Model file for the job. Use its own axes, mm. A direction names the side the tool comes from. Round coordinates to 2 decimals unless told otherwise and drop trailing zeros. Order: outer loops, then holes, each group sorted by start corner. A loop starts at its lowest first (then second) coordinate and runs counter-clockwise, first axis right, second up. Notation, with made-up numbers: (51, 50) - (94, 50) arc R37 ccw to (94, 86) - close; hole circle Ø4 at (44.5, 60). An arc over 180 degrees is marked (long way). Put each result on its own line as item: value. Start each with the question number.
Item 1: Probe probe 1 along Z at (x, y) = (0, 7); probe 2 along Z at (x, y) = (-22.5, 4.5); probe 3 along X at (y, z) = (3, 5). List the from-to ranges inside material, lowest first.
Item 2: Pin check, flat tips, straight feed: pin 1 Ø3 at (y, z) = (4, 2) entering from +X; pin 2 Ø3.5 at (x, y) = (-21, 6) entering from +Z; pin 3 Ø2 at (x, y) = (8.5, 4) entering from -Z. Stop position of each tip, or through.
Item 3: Saw through at A-A on z = 0. List the corners of the cut face in (x, y).
Item 4: Saw through at B-B on y = 3.5. List the corners of the cut face in (x, z).
Item 5: Mould opens along X. For faces 1 (the face through (9.83, 4.93, -37.74)), 2 (the face through (-29, 4, 0)), 3 (the face through (-14, 0, -27)), 4 (the face through (-23.54, 4.44, 16.94)) say: pulls with the +X half, pulls with the -X half, needs draft (parallel to the pull), parting line crosses it, or undercut.
Item 6: Which spindle directions (+Z, -Z, +X, -X, +Y, -Y) get a long thin tool onto all of the face, cutting with end or side? Do faces 5 (the face through (23.54, 4.44, -16.94)), 6 (the face through (9.56, 10.48, -28.94)). Say none if no direction does.
```python
from build123d import *

# Parameters (mm, degrees)
SKETCH1_R           = 39
BOSS_EXTRUDE1_DEPTH = 12
FILLET1_R           = 2
CHAMFER1_SIZE       = 3
SKETCH2_W           = 43
SKETCH2_H           = 43
CUT_EXTRUDE2_DEPTH  = 57.444663167


with BuildPart() as part:
    # Sketch1 → Boss-Extrude1 (new body)
    with BuildSketch(Plane(origin=(0, 0, 0), x_dir=(1, 0, 0), z_dir=(0, 1, 0))):
        with Locations(Location((0, 0, 0), (0, 0, 270))):
            Circle(SKETCH1_R)
        Polygon((17.922985674, 24.668873442), (0, 30.492404503), (-17.922985674, 24.668873442), (-29, 9.422671191), (-29, -9.422671191), (-17.922985674, -24.668873442), (0, -30.492404503), (17.922985674, -24.668873442), (29, -9.422671191), (29, 9.422671191), align=None, mode=Mode.SUBTRACT)
    extrude(amount=BOSS_EXTRUDE1_DEPTH)

    # Fillet1
    fillet1_edges = [part.edges().sort_by_distance(p)[0] for p in [
        (0, 12, -39),
    ]]
    fillet(fillet1_edges, radius=FILLET1_R)

    # Chamfer1
    chamfer1_edges = [part.edges().sort_by_distance(p)[0] for p in [
        (23.461492837, 12, -17.045772316),
        (8.961492837, 12, -27.580638973),
        (-8.961492837, 12, -27.580638973),
        (-23.461492837, 12, -17.045772316),
        (-29, 12, 0),
        (-23.461492837, 12, 17.045772316),
        (-8.961492837, 12, 27.580638973),
        (8.961492837, 12, 27.580638973),
        (23.461492837, 12, 17.045772316),
        (29, 12, 0),
    ]]
    chamfer(chamfer1_edges, length=CHAMFER1_SIZE)

    # Sketch2 → Cut-Extrude2 (cut, through all)
    with BuildSketch(Plane(origin=(0, 0, 0), x_dir=(1, 0, 0), z_dir=(0, 1, 0))):
        with Locations((-7, -47.486840282)):
            Rectangle(SKETCH2_W, SKETCH2_H)
    extrude(amount=CUT_EXTRUDE2_DEPTH, mode=Mode.SUBTRACT)


solid = part.part
```
Results found:
1. probe 1: z = -39 to -30.49
1. probe 2: z = -31.86 to -18.37, 18.37 to 25.99
1. probe 3: x = -38.68 to -29, 29 to 38.68
2. pin 1: stops at x = 39
2. pin 2: stops at z = 25.99
2. pin 3: stops at z = -38.27
3. outline: (-39, 0) - (-29, 0) - (-29, 9) - (-32, 12) - (-37, 12) arc R2 ccw to (-39, 10) - close; (29, 0) - (39, 0) - (39, 10) arc R2 ccw to (37, 12) - (32, 12) - (29, 9) - close
4. outline: (-29, -9.42) - (-29, 9.42) - (-17.92, 24.67) - (-13.87, 25.99) - (-28.5, 25.99) - (-28.5, 26.62) arc R39 ccw (long way) to (14.5, 36.2) - (14.5, 25.99) - (13.87, 25.99) - (17.92, 24.67) - (29, 9.42) - (29, -9.42) - (17.92, -24.67) - (0, -30.49) - (-17.92, -24.67) - close
5. face 1: parting line crosses it
5. face 2: undercut
5. face 3: needs draft
5. face 4: undercut
6. face 5: +Y, -Y
6. face 6: +Y
